```python
from build123d import *
from build123d.topology import SkipClean

# Parameters (mm, degrees)
SKETCH1_R                                       = 7.5
BOSS_EXTRUDE1_DEPTH                             = 10
SKETCH2_W                                       = 95
SKETCH2_H                                       = 75
BOSS_EXTRUDE2_DEPTH                             = 10
LPATTERN1_COUNT                                 = 2
LPATTERN1_PITCH                                 = 85
CUT_EXTRUDE2_DEPTH                              = 77
CUT_EXTRUDE2_DEPTH_BACK                         = 2
SKETCH5_R                                       = 7.5
SKETCH5_R_2                                     = 1
BOSS_EXTRUDE4_DEPTH                             = 10
CSK_FOR_M3_FLAT_HEAD_MACHINE_SCREW1_D           = 3.4
CSK_FOR_M3_FLAT_HEAD_MACHINE_SCREW1_DEPTH       = 95
CSK_FOR_M3_FLAT_HEAD_MACHINE_SCREW1_CSINK_D     = 6.3
CSK_FOR_M3_FLAT_HEAD_MACHINE_SCREW1_CSINK_ANGLE = 90
BOSS_EXTRUDE5_START                             = -10
SKETCH10_R                                      = 7.5
BOSS_EXTRUDE5_DEPTH                             = 10


with BuildPart() as part:
    # Sketch1 → Boss-Extrude1 (new body)
    with BuildSketch(Plane.YZ):
        with BuildLine():
            Line((-14.116239718, 5.072649824), (-37.5, -60))
            Line((-37.5, -60), (37.5, -60))
            Line((37.5, -60), (14.116239718, 5.072649824))
            ThreePointArc((14.116239718, 5.072649824), (0, 15), (-14.116239718, 5.072649824))
        make_face()
        with Locations(Location((0, 0, 0), (0, 0, 270))):
            Circle(SKETCH1_R, mode=Mode.SUBTRACT)
    boss_extrude1 = extrude(amount=BOSS_EXTRUDE1_DEPTH)

    # Sketch2 → Boss-Extrude2 (add)
    with BuildSketch(Plane(origin=(0, 0, -60), x_dir=(1, 0, 0), z_dir=(0, 0, -1))):
        with Locations((47.5, 0)):
            Rectangle(SKETCH2_W, SKETCH2_H)
    extrude(amount=BOSS_EXTRUDE2_DEPTH)

    # LPattern1: Boss-Extrude1 ×2
    with Locations(*[(i * LPATTERN1_PITCH, 0, 0) for i in range(1, LPATTERN1_COUNT)]):
        add(boss_extrude1)

    # Sketch4 → Cut-Extrude2 (cut, two sides: drawn at the far end of the back side and taken through both)
    with SkipClean():  # the faces are left unmerged after this step: merging them gives an invalid solid
        with BuildSketch(Plane.YZ.offset(10).offset(-CUT_EXTRUDE2_DEPTH_BACK)):
            with BuildLine():
                Line((-37.5, -60), (37.5, -60))
                Line((37.5, -60), (14.116239718, 5.072649824))
                ThreePointArc((14.116239718, 5.072649824), (14.777408362, 2.574529494), (15, 0))
                ThreePointArc((15, 0), (-2.574529494, -14.777408362), (-14.116239718, 5.072649824))
                Line((-14.116239718, 5.072649824), (-37.5, -60))
            make_face()
        extrude(amount=CUT_EXTRUDE2_DEPTH + CUT_EXTRUDE2_DEPTH_BACK, mode=Mode.SUBTRACT)

    # Sketch5 → Boss-Extrude4 (add)
    with SkipClean():  # the faces are left unmerged after this step: merging them gives an invalid solid
        with BuildSketch(Plane.YZ):
            with Locations(Location((0, 0, 0), (0, 0, 270))):
                Circle(SKETCH5_R)
            with Locations(Location((0, 0, 0), (0, 0, 270))):
                Circle(SKETCH5_R_2, mode=Mode.SUBTRACT)
        extrude(amount=BOSS_EXTRUDE4_DEPTH)

    # CSK for M3 Flat Head Machine Screw1
    with Locations(Plane(origin=(0, 0, 0), x_dir=(0, -1, 0), z_dir=(-1, 0, 0))):
        with Locations((0, 0)):
            CounterSinkHole(CSK_FOR_M3_FLAT_HEAD_MACHINE_SCREW1_D / 2, CSK_FOR_M3_FLAT_HEAD_MACHINE_SCREW1_CSINK_D / 2, depth=CSK_FOR_M3_FLAT_HEAD_MACHINE_SCREW1_DEPTH, counter_sink_angle=CSK_FOR_M3_FLAT_HEAD_MACHINE_SCREW1_CSINK_ANGLE)

    # Sketch10 → Boss-Extrude5 (add)
    with SkipClean():  # the faces are left unmerged after this step: merging them gives an invalid solid
        with BuildSketch(Plane.YZ.offset(95).offset(BOSS_EXTRUDE5_START)):
            Circle(SKETCH10_R)
            with BuildLine():
                Line((-3.5, -3.570714214), (3.5, -3.570714214))
                ThreePointArc((3.5, -3.570714214), (0, 5), (-3.5, -3.570714214))
            make_face(mode=Mode.SUBTRACT)
        extrude(amount=BOSS_EXTRUDE5_DEPTH)


solid = part.part
```
Geometry: final body of the model. Coordinates: model frame, mm. A direction names the side the tool comes from. Coordinates: 2 decimals unless noted, no trailing zeros. Write each loop counter-clockwise with the first axis right and the second up, starting at its lowest first coordinate (ties: lowest second). Pieces come first, ordered by that corner, then holes. Notation, with made-up numbers: M 51,-26 L 57,-26 A34 cw 57,4 Z; hole C 6.5,-21.5 d7. An arc over 180 degrees is marked long. Use CSV: the item, a comma, the result in double quotes. Start each with the question number.
1. First-contact query: P1, Ø4, axis at y = 0, z = 0, coming from the +X side; P2, Ø19.5, axis at y = -6, z = -18, coming from the -X side; P3, Ø22.5, axis at x = 58.5, y = 3.5, coming from the +Z side; P4, Ø5, axis at x = 83.5, z = 4.5, coming from the +Y side. Flat tips, straight axial feed; report the tip coordinate or a pass-through.
2. Reachability of faces 1 (the face through (85, -4, 4)), 2 (the face through (90, 0, -3.571)), 3 (the face through (91, 26, -28)) from +Z, -Z, +X, -X, +Y, -Y: full face, straight path, thin tool, end or side. Return the list, or none.
3. Cut plane A-A on y = 0. Return the cut outline in (x, z), plus the area to 3 significant figures.
4. Mould query, pull axis X, two halves, no side actions, for faces 4 (the face through (95, -1, -36)), 5 (the face through (87, -1, -34)), 6 (the face through (47, -1, -60)), 7 (the face through (3.944, -25.644, -27.008)). Classes: pulls with the +X half, pulls with the -X half, needs draft (parallel to the pull), parting line crosses it, or undercut.
5. Cut plane C-C on x = 26.5. Return the cut outline in (y, z), plus the area to 3 significant figures.
6. Ray query, probe 1 along X at (y, z) = (-10, -54.5); probe 2 along Y at (x, z) = (88.5, 0); probe 3 along Y at (x, z) = (7, 0). Return the intervals inside material, ascending.
7. Cut plane B-B on z = -43.5. Return the cut outline in (x, y), plus the area to 3 significant figures.
8. Cut plane D-D on y = 21.5. Return the cut outline in (x, z).
Entries:
1,P1,"x = 10"
1,P2,"x = 0"
1,P3,"z = -60"
1,P4,"y = 14.79"
2,face 1,"+Z, +Y, -Y"
2,face 2,"+X"
2,face 3,"+Z, +X, -X, +Y"
3,outline,"M 0,-70 L 95,-70 L 95,-3.57 L 85,-3.57 L 85,-15 L 87,-15 L 87,-60 L 8,-60 L 8,-15 L 10,-15 L 10,-1.7 L 1.45,-1.7 L 0,-3.15 Z; M 0,3.15 L 1.45,1.7 L 10,1.7 L 10,15 L 0,15 Z; M 85,5 L 95,5 L 95,15 L 85,15 Z"
3,area,"2,150 mm²"
4,face 4,"pulls with the +X half"
4,face 5,"undercut"
4,face 6,"undercut"
4,face 7,"needs draft"
5,outline,"M -37.5,-70 L 37.5,-70 L 37.5,-60 L -37.5,-60 Z"
5,area,"750 mm²"
6,probe 1,"0 to 8, 87 to 95"
6,probe 2,"-15.94 to -5, 5 to 15.94"
6,probe 3,"-15.94 to -1.7, 1.7 to 15.94"
7,outline,"M 0,-31.57 L 8,-31.57 L 8,31.57 L 0,31.57 Z; M 87,-31.57 L 95,-31.57 L 95,31.57 L 87,31.57 Z"
7,area,"1,010 mm²"
8,outline,"M 0,-70 L 95,-70 L 95,-15.47 L 87,-15.47 L 87,-60 L 8,-60 L 8,-15.47 L 0,-15.47 Z"
